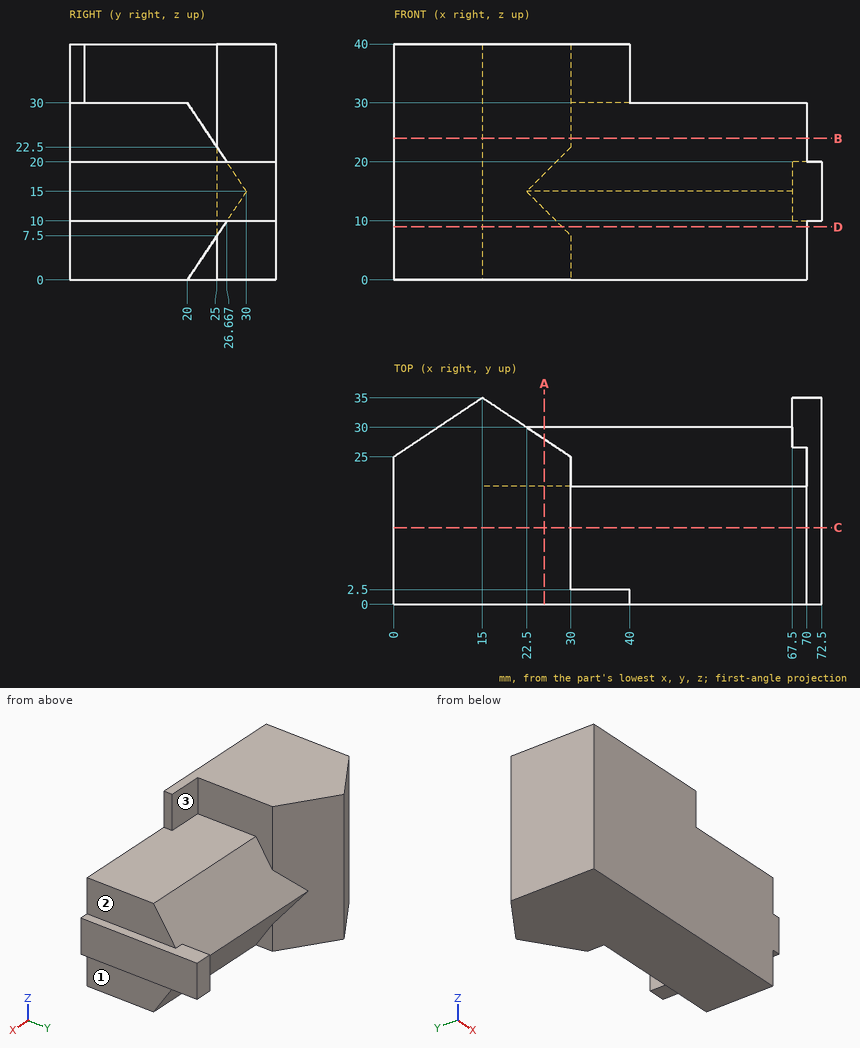
Geometry check sheet. Reference: drawing and pictorial views, mm from the part's lowest x, y, z. A direction names the side the tool comes from. Coordinates: 2 decimals unless noted, no trailing zeros. Loops run counter-clockwise (first coordinate to the right, second up) from the corner with the lowest first, then second, coordinate; pieces in that order, holes last. Notation, with made-up numbers: (-36.75, 39.25) -> (-31.75, 39.25) arc R11 cw to (-31.75, 58.25) -> close; hole circle Ø1 at (71, 79.5). An arc over 180 degrees is marked (long way). Put each result on its own line as item: value.
1) Thickness scan on line 1 (Z direction, x = 49, y = 4.5); line 2 (Y direction, x = 27.5, z = 31). Record the ranges inside material, lowest first.
Result set:
line 1: z = 0 to 30
line 2: y = 0 to 26.67
2) Cross-section at B-B on z = 24. Record the boundary of the cut face in (x, y).
Result set:
outline: (0, 0) -> (70, 0) -> (70, 24) -> (30, 24) -> (30, 25) -> (15, 35) -> (0, 25) -> close
3) Cross-section at C-C on y = 13. Record the boundary of the cut face in (x, z), plus the area to 4 significant figures.
Result set:
outline: (0, 0) -> (70, 0) -> (70, 10) -> (72.5, 10) -> (72.5, 20) -> (70, 20) -> (70, 30) -> (30, 30) -> (30, 40) -> (0, 40) -> close
area: 2,425 mm^2
4) Gauge pin test, flat ends, axial feed: pin 1 Ø10 at (y, z) = (31, 4) entering from -X; pin 2 Ø14 at (y, z) = (16.5, 33) entering from +X; pin 3 Ø6 at (y, z) = (26.5, 29) entering from +X. Record the tip position at first contact, or that the pin passes through.
Result set:
pin 1: stops at x = 1.5
pin 2: stops at x = 70
pin 3: stops at x = 30
5) Cross-section at A-A on x = 25.5. Record the boundary of the cut face in (y, z).
Result set:
outline: (0, 0) -> (28, 0) -> (28, 12) -> (30, 15) -> (28, 18) -> (28, 40) -> (0, 40) -> close
6) Cross-section at D-D on z = 9. Record the boundary of the cut face in (x, y).
Result set:
outline: (0, 0) -> (70, 0) -> (70, 26) -> (28.5, 26) -> (15, 35) -> (0, 25) -> close
7) Tool access check on the marked faces 1, 2 and 3. Record the directions out of +Z, -Z, +X, -X, +Y, -Y that give a thin tool (end or side, any length) a straight path to the whole face; none if there is none.
Result set:
face 1: -Z, +X, +Y, -Y
face 2: +Z, +X, +Y, -Y
face 3: +Z, +X, +Y
